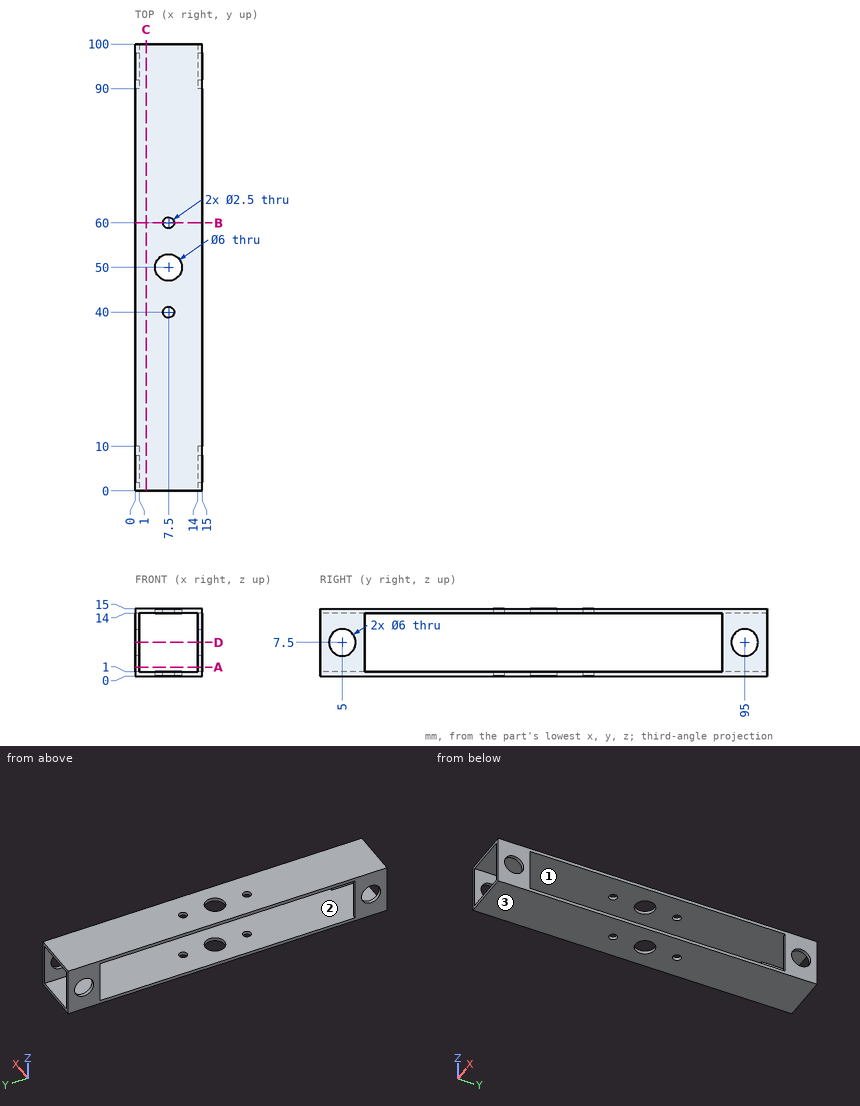
Print and shaded views of the part. All mm, measured from the part's lowest x, y and z. Coordinates: 2 decimals unless noted, no trailing zeros. Loops run counter-clockwise (first coordinate to the right, second up) from the corner with the lowest first, then second, coordinate; pieces in that order, holes last. Notation, with made-up numbers: (75.5, -5) - (115.5, -5) arc R29 ccw to (115.5, 23) - close; hole circle Ø6 at (23.5, -13.75). An arc over 180 degrees is marked (long way). Write item = value, one per line. Start each with the question number.
Item 1: Saw through at A-A, the plane z = 2. List the corners of the cut face in (x, y).
Item 2: Saw through at C-C, the plane x = 2.5. List the corners of the cut face in (y, z), then the cut area to 3 significant figures.
Item 3: Pull direction X, two halves, no side cores. Call the marked faces 1, 2 and 3: +X half, -X half, draft (parallel to the pull), parting line (faces both ways), or undercut.
Item 4: Saw through at B-B, the plane y = 60. List the corners of the cut face in (x, z), then the cut area to 3 significant figures.
Item 5: Wall check: probe 1 along Y at (x, z) = (7.5, 14.6); probe 2 along Y at (x, z) = (0.85, 7.5); probe 3 along X at (y, z) = (7.5, 12). Give the ranges that are in metal, low to high. Write a range as [from, to].
Item 6: Saw through at D-D, the plane z = 7.5. State how many separate pieces and enclosed holes the cut face has, then the cut area to 3 significant figures.
Item 7: Drop a flat-ended pin along its axis: pin 1 Ø3 at (y, z) = (21, 12) entering from -X. Give the stop position or say it passes through.
Answers:
q1.outline = (0, 0) - (1, 0) - (1, 10) - (0, 10) - close; (0, 90) - (1, 90) - (1, 100) - (0, 100) - close; (14, 0) - (15, 0) - (15, 10) - (14, 10) - close; (14, 90) - (15, 90) - (15, 100) - (14, 100) - close
q2.outline = (0, 0) - (100, 0) - (100, 1) - (0, 1) - close; (0, 14) - (100, 14) - (100, 15) - (0, 15) - close
q2.area = 200 mm2
q3.face_1 = undercut
q3.face_2 = undercut
q3.face_3 = draft
q4.outline = (0, 0) - (6.25, 0) - (6.25, 1) - (0, 1) - close; (0, 14) - (6.25, 14) - (6.25, 15) - (0, 15) - close; (8.75, 0) - (15, 0) - (15, 1) - (8.75, 1) - close; (8.75, 14) - (15, 14) - (15, 15) - (8.75, 15) - close
q4.area = 25.0 mm2
q5.probe_1 = [0, 38.75], [41.25, 47], [53, 58.75], [61.25, 100]
q5.probe_2 = [0, 2], [8, 10], [90, 92], [98, 100]
q5.probe_3 = [0, 1], [14, 15]
q6.separate_pieces = 8
q6.enclosed_holes = 0
q6.area = 16.0 mm2
q7.pin_1 = through
